Work out the finished part from the listing and answer in its coordinate system (mm). Face numbers are marked on the shaded views. A direction names the side the tool comes from. Coordinates: 2 decimals unless noted, no trailing zeros. Order: outer loops, then holes, each group sorted by start corner. A loop starts at its lowest first (then second) coordinate and runs counter-clockwise, first axis right, second up. Notation, with made-up numbers: M 85.5,40.5 L 112.5,40.5 A26 cw 112.5,64.5 Z; hole C -4,71.25 d5. An arc over 180 degrees is marked long. Use a Markdown table: item, result.
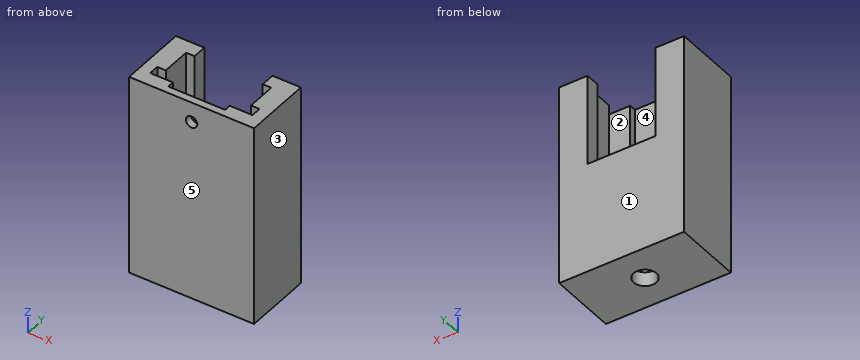
from build123d import *

# Parameters (mm, degrees)
F0_W     = 27.94
F0_H     = 15.24
F0_R     = 2.54
F1_DEPTH = 3.175
F2_W     = 27.94
F2_H     = 15.24
F2_W_2   = 19.05
F2_H_2   = 8.89
F3_DEPTH = 10.16
F4_W     = 27.94
F4_H     = 15.24
F5_DEPTH = 31.75
F6_W     = 15.24
F6_H     = 3.175
F7_DEPTH = 20.32
F8_R     = 1.27
F9_DEPTH = 1.651


with BuildPart() as f1:
    # F0 (on Top) → F1 (new body)
    with BuildSketch(Plane.XY):
        Rectangle(F0_W, F0_H)
        Circle(F0_R, mode=Mode.SUBTRACT)
    extrude(amount=F1_DEPTH)

    # F2 (on face) → F3 (join)
    with BuildSketch(Plane.XY.offset(3.175)):
        Rectangle(F2_W, F2_H)
        Rectangle(F2_W_2, F2_H_2, mode=Mode.SUBTRACT)
    extrude(amount=F3_DEPTH)

    # F4 (on face) → F5 (join)
    with BuildSketch(Plane.XY.offset(13.335)):
        Rectangle(F4_W, F4_H)
        Polygon((-9.525, -4.445), (-11.43, -4.445), (-11.43, -2.159), (-9.525, -2.159), (-9.525, 4.445), (9.525, 4.445), (9.525, -2.159), (11.43, -2.159), (11.43, -4.445), (9.525, -4.445), (6.35, -4.445), (6.35, -5.969), (-6.35, -5.969), (-6.35, -4.445), align=None, mode=Mode.SUBTRACT)
    extrude(amount=F5_DEPTH)

    # F6 (on face) → F7 (cut)
    with BuildSketch(Plane.XY.offset(45.085)):
        with Locations((0, 6.0325)):
            Rectangle(F6_W, F6_H)
    extrude(amount=-F7_DEPTH, mode=Mode.SUBTRACT)

    # F8 (on face) → F9 (cut, through all)
    with BuildSketch(Plane(origin=(0, -5.969, 0), x_dir=(-1, 0, 0), z_dir=(0, 1, 0))):
        with Locations((0, 40.6052581966)):
            Circle(F8_R)
    extrude(amount=-F9_DEPTH, mode=Mode.SUBTRACT)


solid = f1.part
(1) A cutting plane is placed at D-D (z = 33). Determine the outline of the cut face in (x, y) (3 decimals), then the cut area to 3 significant figures.
Conclusion:
| item | result |
|---|---|
| outline | M -13.97,-7.62 L 13.97,-7.62 L 13.97,7.62 L 7.62,7.62 L 7.62,4.445 L 9.525,4.445 L 9.525,-2.159 L 11.43,-2.159 L 11.43,-4.445 L 6.35,-4.445 L 6.35,-5.969 L -6.35,-5.969 L -6.35,-4.445 L -11.43,-4.445 L -11.43,-2.159 L -9.525,-2.159 L -9.525,4.445 L -7.62,4.445 L -7.62,7.62 L -13.97,7.62 Z |
| area | 180 mm2 |
(2) A cutting plane is placed at C-C (z = 6). Determine the outline of the cut face in (x, y) (3 decimals), then the cut area to 3 significant figures.
Conclusion:
| item | result |
|---|---|
| outline | M -13.97,-7.62 L 13.97,-7.62 L 13.97,7.62 L -13.97,7.62 Z; hole M -9.525,-4.445 L 9.525,-4.445 L 9.525,4.445 L -9.525,4.445 Z |
| area | 256 mm2 |
(3) Straight lines are drawn through the part: L1, parallel to X at y = 0.25, z = 17.5 (3 decimals); L2, parallel to X at y = -3.5, z = 33.5; L3, parallel to Y at x = 0, z = 1.8. For each, find the intervals that lie inside material, in ascending order.
Conclusion:
| item | result |
|---|---|
| L1 | -13.97 to -9.525, 9.525 to 13.97 |
| L2 | -13.97 to -11.43, 11.43 to 13.97 |
| L3 | -7.62 to -2.54, 2.54 to 7.62 |
(4) A cutting plane is placed at B-B (y = 0). Determine the outline of the cut face in (x, z) (3 decimals), then the cut area to 3 significant figures.
Conclusion:
| item | result |
|---|---|
| outline | M -13.97,0 L -2.54,0 L -2.54,3.175 L -9.525,3.175 L -9.525,45.085 L -13.97,45.085 Z; M 2.54,0 L 13.97,0 L 13.97,45.085 L 9.525,45.085 L 9.525,3.175 L 2.54,3.175 Z |
| area | 445 mm2 |
(5) Given P1, Ø3.5, axis at x = 2, y = 6.5, coming from the +Z side (3 decimals); P2, Ø1.5, axis at x = -3, y = -1.5, coming from the +Z side (3 decimals); P3, Ø0.6, axis at x = 11, y = -3.5, coming from the +Z side (3 decimals), each flat-ended and moving along its own axis, determine where each tip first touches the part or whether it passes through.
Conclusion:
| item | result |
|---|---|
| P1 | z = 24.765 |
| P2 | z = 3.175 |
| P3 | z = 13.335 |
(6) Determine the mould class of the marked faces 1, 2 and 3 for opening direction X: pulls with the +X half, pulls with the -X half, needs draft (parallel to the pull), parting line crosses it, or undercut.
Conclusion:
| item | result |
|---|---|
| face 1 | needs draft |
| face 2 | undercut |
| face 3 | pulls with the +X half |
(7) A cutting plane is placed at A-A (x = 0). Determine the outline of the cut face in (y, z) (3 decimals).
Conclusion:
| item | result |
|---|---|
| outline | M -7.62,0 L -2.54,0 L -2.54,3.175 L -4.445,3.175 L -4.445,13.335 L -5.969,13.335 L -5.969,39.335 L -7.62,39.335 Z; M -7.62,41.875 L -5.969,41.875 L -5.969,45.085 L -7.62,45.085 Z; M 2.54,0 L 7.62,0 L 7.62,24.765 L 4.445,24.765 L 4.445,3.175 L 2.54,3.175 Z |
(8) Which of the six approach directions +Z, -Z, +X, -X, +Y, -Y give full straight-line access (tool end or side, diameter ignored) to the marked faces 4 and 5?
Conclusion:
| item | result |
|---|---|
| face 4 | +Z |
| face 5 | +Z, -Z, +X, -X, -Y |
